Source: CAD feature listing. Evaluate the final solid. Frame: model axes, mm. Face numbers are marked on the shaded views. A direction names the side the tool comes from. Coordinates: 2 decimals unless noted, no trailing zeros. Write each loop counter-clockwise with the first axis right and the second up, starting at its lowest first coordinate (ties: lowest second). Pieces come first, ordered by that corner, then holes. Notation, with made-up numbers: M 2.25,69.25 L 40.25,69.25 A13 cw 40.25,86.25 Z; hole C -10,9 d1. An arc over 180 degrees is marked long. One line per item, written item: value. Start each with the question number.
Item 1: Mould query, pull axis X, two halves, no side actions, for the marked faces 3, 4 and 5. Classes: released by +X, released by -X, zero draft, split by the parting line, or undercut.
Item 2: Cut plane A-A, the plane z = 11. Output: boundary loops of the cut face in (x, y).
Item 3: Cut plane C-C, the plane x = 38. Output: boundary loops of the cut face in (y, z), then the cut area to 3 significant figures.
Item 4: Cut plane B-B, the plane y = 24.5. Output: boundary loops of the cut face in (x, z), then the cut area to 3 significant figures.
Item 5: Ray query, L1, parallel to X at y = 31.5, z = 6.25; L2, parallel to Y at x = 41, z = 13; L3, parallel to Z at x = 33.5, y = 15.5. Return the intervals inside material, ascending. Write a range as from..to.
Item 6: Pin query (flat end, axial travel): P1, Ø23, axis at x = 21, y = 18.5, coming from the +Z side. Return the tip coordinate at first contact, or that it passes through.
Item 7: Set-up query: the marked faces 1 and 2. Return all of +Z, -Z, +X, -X, +Y, -Y with unobstructed straight access to the full face (end or side cutting, diameter ignored); none if empty.
Autodesk Fusion 360 part; units mm, degrees
sketch "Skizze1" plane through (0, 0, 0) normal (0, 0, 1) x (1, 0, 0)
  line L0 (0, 0) -> (60, 0)
  line L1 (60, 0) -> (60, 50)
  line L2 (60, 50) -> (0, 50)
  line L3 (0, 50) -> (0, 0)
  dimension "d1" = 60
  dimension "d2" = 50
extrude "Extrusion1" add sketch "Skizze1" along normal blind 5
sketch "Skizze2" plane through (0, 0, 5) normal (0, 0, 1) x (-1, 0, 0)
  line L0 (0, -50) -> (0, 0)
  line L1 (0, 0) -> (-60, 0)
  line L2 (-60, 0) -> (-60, -50)
  line L3 (-60, -50) -> (0, -50)
  line L4 (-58, -2) -> (-58, -48)
  line L5 (-58, -48) -> (-2, -48)
  line L6 (-2, -48) -> (-2, -2)
  line L7 (-2, -2) -> (-58, -2)
  dimension "d5" = -2
extrude "Extrusion2" add sketch "Skizze2" along normal blind 10
scale "Maßstab1" factor 1 about (60, 0, 0) bodies 1
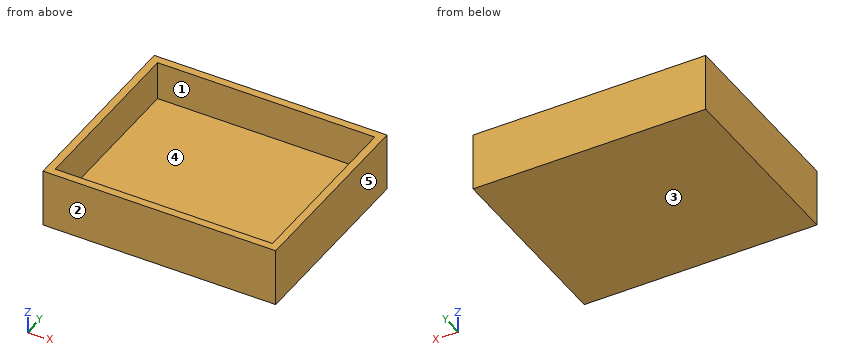
From the geometry:
1. face 3: zero draft
1. face 4: undercut
1. face 5: released by +X
2. outline: M 0,0 L 60,0 L 60,50 L 0,50 Z; hole M 2,2 L 58,2 L 58,48 L 2,48 Z
3. outline: M 0,0 L 50,0 L 50,15 L 48,15 L 48,5 L 2,5 L 2,15 L 0,15 Z
3. area: 290 mm²
4. outline: M 0,0 L 60,0 L 60,15 L 58,15 L 58,5 L 2,5 L 2,15 L 0,15 Z
4. area: 340 mm²
5. L1: x = 0..2, 58..60
5. L2: y = 0..2, 48..50
5. L3: z = 0..5
6. P1: stops at z = 5
7. face 1: +Z
7. face 2: +Z, -Z, +X, -X, -Y
